```python
from build123d import *

# Parameters (mm, degrees)
SKETCH1_R                                     = 57.5
SKETCH1_R_2                                   = 0.5
SKETCH1_W                                     = 9.325
SKETCH1_H                                     = 9.9
BOSS_EXTRUDE1_DEPTH                           = 3
CSK_FOR_8_FLAT_HEAD_SOCKET_CAP_SCREW1_A_COUNT = 2
CSK_FOR_8_FLAT_HEAD_SOCKET_CAP_SCREW1_A_PITCH = 67.882250994
CSK_FOR_8_FLAT_HEAD_SOCKET_CAP_SCRE_2_COUNT   = 2
CSK_FOR_8_FLAT_HEAD_SOCKET_CAP_SCRE_2_PITCH   = 96
CSK_FOR_8_FLAT_HEAD_SOCKET_CAP_SCRE_3_COUNT   = 2
CSK_FOR_8_FLAT_HEAD_SOCKET_CAP_SCRE_3_PITCH   = 67.882250994
SKETCH5_W                                     = 4.075
SKETCH5_H                                     = 9.9
CUT_EXTRUDE2_DEPTH                            = 4
CUT_EXTRUDE4_DEPTH                            = 4
FILLET3_R                                     = 2


with BuildPart() as part:
    # Sketch1 → Boss-Extrude1 (new body)
    with BuildSketch(Plane(origin=(0, 0, 0), x_dir=(1, 0, 0), z_dir=(0, 1, 0))):
        Circle(SKETCH1_R)
        with Locations((-33.941125497, 33.941125497)):
            Circle(SKETCH1_R_2, mode=Mode.SUBTRACT)
        with Locations((33.941125497, 33.941125497)):
            Circle(SKETCH1_R_2, mode=Mode.SUBTRACT)
        with Locations((33.941125497, -33.941125497)):
            Circle(SKETCH1_R_2, mode=Mode.SUBTRACT)
        with Locations((-33.941125497, -33.941125497)):
            Circle(SKETCH1_R_2, mode=Mode.SUBTRACT)
        with Locations((1.6625, 0)):
            Rectangle(SKETCH1_W, SKETCH1_H, mode=Mode.SUBTRACT)
    extrude(amount=BOSS_EXTRUDE1_DEPTH)

    # Sketch2 → CSK for #8 Flat Head Socket Cap Screw1 (revolve, cut)
    with BuildSketch(Plane(origin=(-33.941125497, 0, 33.941125497), x_dir=(0, 0, -1), z_dir=(1, 0, 0))):
        Polygon((0, 0), (0, 3), (2.45745, 3), (2.45745, 2.417901837), (4.5593, 0), align=None)
    csk_for_8_flat_head_socket_cap_screw1 = revolve(axis=Axis((-33.941125497, -6.35, 33.941125497), (0, 1, 0)), mode=Mode.SUBTRACT)

    # CSK for #8 Flat Head Socket Cap Screw1 a: CSK for #8 Flat Head Socket Cap Screw1 ×2
    with Locations(*[(i * CSK_FOR_8_FLAT_HEAD_SOCKET_CAP_SCREW1_A_PITCH, 0, 0) for i in range(1, CSK_FOR_8_FLAT_HEAD_SOCKET_CAP_SCREW1_A_COUNT)]):
        add(csk_for_8_flat_head_socket_cap_screw1, mode=Mode.SUBTRACT)

    # CSK for _8 Flat Head Socket Cap Scre 2: CSK for #8 Flat Head Socket Cap Screw1 ×2
    with Locations(*[Vector(0.707106781, 0, -0.707106781) * (i * CSK_FOR_8_FLAT_HEAD_SOCKET_CAP_SCRE_2_PITCH) for i in range(1, CSK_FOR_8_FLAT_HEAD_SOCKET_CAP_SCRE_2_COUNT)]):
        add(csk_for_8_flat_head_socket_cap_screw1, mode=Mode.SUBTRACT)

    # CSK for _8 Flat Head Socket Cap Scre 3: CSK for #8 Flat Head Socket Cap Screw1 ×2
    with Locations(*[(0, 0, -i * CSK_FOR_8_FLAT_HEAD_SOCKET_CAP_SCRE_3_PITCH) for i in range(1, CSK_FOR_8_FLAT_HEAD_SOCKET_CAP_SCRE_3_COUNT)]):
        add(csk_for_8_flat_head_socket_cap_screw1, mode=Mode.SUBTRACT)

    # Sketch5 → Cut-Extrude2 (cut, through all)
    with BuildSketch(Plane.XZ):
        with Locations((8.3625, 0)):
            Rectangle(SKETCH5_W, SKETCH5_H)
        with Locations((-5.0375, 0)):
            Rectangle(SKETCH5_W, SKETCH5_H)
    extrude(amount=-CUT_EXTRUDE2_DEPTH, mode=Mode.SUBTRACT)

    # Sketch10 → Cut-Extrude4 (cut, through all)
    with BuildSketch(Plane.XZ):
        with BuildLine():
            Line((23.40393029, 36.072926787), (10.885548972, 16.778105482))
            ThreePointArc((10.885548972, 16.778105482), (0, 20), (-10.885548972, 16.778105482))
            Line((-10.885548972, 16.778105482), (-23.40393029, 36.072926787))
            ThreePointArc((-23.40393029, 36.072926787), (0, 43), (23.40393029, 36.072926787))
        make_face()
        with BuildLine():
            Line((-23.40393029, -36.072926787), (-10.885548972, -16.778105482))
            ThreePointArc((-10.885548972, -16.778105482), (0, -20), (10.885548972, -16.778105482))
            Line((10.885548972, -16.778105482), (23.40393029, -36.072926787))
            ThreePointArc((23.40393029, -36.072926787), (0, -43), (-23.40393029, -36.072926787))
        make_face()
    extrude(amount=-CUT_EXTRUDE4_DEPTH, mode=Mode.SUBTRACT)

    # Fillet3
    fillet3_edges = [part.edges().sort_by_distance(p)[0] for p in [
        (10.885548972, 1.5, 16.778105482),
        (-10.885548972, 1.5, 16.778105482),
        (-10.885548972, 1.5, -16.778105482),
        (10.885548972, 1.5, -16.778105482),
        (23.40393029, 1.5, -36.072926787),
        (-23.40393029, 1.5, -36.072926787),
        (-23.40393029, 1.5, 36.072926787),
        (23.40393029, 1.5, 36.072926787),
    ]]
    fillet(fillet3_edges, radius=FILLET3_R)


solid = part.part
```
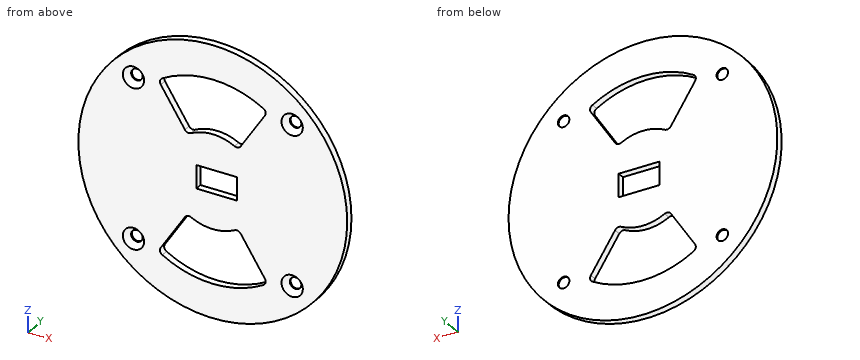
CAD build for the part. Positions are in the model's coordinates, mm. Coordinates: 2 decimals unless noted, no trailing zeros. Order: outer loops, then holes, each group sorted by start corner. A loop starts at its lowest first (then second) coordinate and runs counter-clockwise, first axis right, second up. Notation, with made-up numbers: (21, 39) - (40, 39) arc R29 cw to (40, 64) - close; hole circle Ø8 at (-13, -14.75). An arc over 180 degrees is marked (long way). Use a Markdown table: item, result. Add a question column.
(1) Saw through at D-D (z = 28). Give the cut face in (x, y).
(2) Flat gauge pins, fed straight in: pin 1 (4 mm diameter, centred on x = -26.5, z = 13.5, fed in from -Y); pin 2 (1 mm diameter, centred on y = 2.5, z = -24, fed in from -X); pin 3 (1.5 mm diameter, centred on y = 0.5, z = -43, fed in from -X); pin 4 (1 mm diameter, centred on x = -35, y = 1, fed in from -Z). Where does each tip first touch, or does it go through?
(3) Drill centre lines: line 1 along Z through (x, y) = (-0.5, 2.15); line 2 along Z through (x, y) = (18, 2.7); line 3 along Z through (x, y) = (10.5, 0.75). Where is each one in solid material? Low to high. Write a range as [from, to].
(4) Saw through at C-C (y = 0.55). Count the separate pieces of the cut face and the enclosed holes in it, then the cut area to 3 significant figures.
(5) Saw through at B-B (z = -26). Give the cut face in (x, y).
(6) Saw through at A-A (x = 0). Give the cut face in (y, z), then the cut area to 3 significant figures.
Solved:
| question | item | result |
|---|---|---|
| 1 | outline | (-50.22, 0) - (-18.17, 0) - (-18.17, 3) - (-50.22, 3) - close; (18.17, 0) - (50.22, 0) - (50.22, 3) - (18.17, 3) - close |
| 2 | pin 1 | stops at y = 0 |
| 2 | pin 2 | stops at x = -52.48 |
| 2 | pin 3 | stops at x = -39 |
| 2 | pin 4 | stops at z = -46 |
| 3 | line 1 | z = [-57.5, -43], [-19.99, -4.95], [4.95, 19.99], [43, 57.5] |
| 3 | line 2 | z = [-54.61, -39.05], [-27.74, 27.74], [39.05, 54.61] |
| 3 | line 3 | z = [-56.53, -41.7], [-17.48, 17.48], [41.7, 56.53] |
| 4 | separate pieces | 1 |
| 4 | enclosed holes | 7 |
| 4 | area | 8,340 mm² |
| 5 | outline | (-51.29, 0) - (-16.87, 0) - (-16.87, 3) - (-51.29, 3) - close; (16.87, 0) - (51.29, 0) - (51.29, 3) - (16.87, 3) - close |
| 6 | outline | (0, -57.5) - (3, -57.5) - (3, -43) - (0, -43) - close; (0, -20) - (3, -20) - (3, -4.95) - (0, -4.95) - close; (0, 4.95) - (3, 4.95) - (3, 20) - (0, 20) - close; (0, 43) - (3, 43) - (3, 57.5) - (0, 57.5) - close |
| 6 | area | 177 mm² |
